Autodesk Inventor part; units mm, degrees
ref_plane "YZ Plane" through (0, 0, 0) normal (1, 0, 0) x (0, 1, 0)
ref_plane "XZ Plane" through (0, 0, 0) normal (0, 1, 0) x (-1, 0, 0)
ref_plane "XY Plane" through (0, 0, 0) normal (0, 0, 1) x (1, 0, 0)
sketch "Base" plane through (0, 0, 0) normal (0, 0, 1) x (1, 0, 0)
  circle A0 centre (0, 0) radius 19.125 construction
  arc A1 (28.5, 24.5) -> (24.5, 28.5) centre (24.5, 24.5) ccw
  line L0 (24.5, 28.5) -> (-24.5, 28.5)
  arc A2 (-24.5, 28.5) -> (-28.5, 24.5) centre (-24.5, 24.5) ccw
  line L1 (-28.5, 24.5) -> (-28.5, -24.5)
  arc A3 (-28.5, -24.5) -> (-24.5, -28.5) centre (-24.5, -24.5) ccw
  line L2 (-24.5, -28.5) -> (24.5, -28.5)
  arc A4 (24.5, -28.5) -> (28.5, -24.5) centre (24.5, -24.5) ccw
  line L3 (28.5, -24.5) -> (28.5, 24.5)
  circle A5 centre (-23.57, 23.57) radius 2
  circle A6 centre (23.57, 23.57) radius 2
  circle A7 centre (-23.57, -23.57) radius 2
  circle A8 centre (23.57, -23.57) radius 2
  circle A9 centre (0, 0) radius 20.125
  circle A10 centre (-17.9605, 17.9605) radius 2.489
  circle A11 centre (17.9605, -17.9605) radius 2.489
  point P0 (0, 0)
  dimension "d0" = 1
extrude "Plate1" add sketch "Base" along normal blind 2.54
sketch "Sketch2" plane through (0, 0, 2.54) normal (0, 0, 1) x (1, 0, 0)
  line L0 (28.5, -24.5) -> (28.5, 24.5)
  line L1 (28.5, -24.5) -> (28.5, -84.5)
  line L2 (-28.5, 24.5) -> (-28.5, -24.5)
  line L3 (-28.5, -24.5) -> (-28.5, -84.5)
  line L4 (28.5, -84.5) -> (-28.5, -84.5)
  arc A0 (24.5, -28.5) -> (28.5, -24.5) centre (24.5, -24.5) ccw
  line L5 (24.5, -28.5) -> (-24.5, -28.5)
  arc A1 (-28.5, -24.5) -> (-24.5, -28.5) centre (-24.5, -24.5) ccw
  point P0 (0, 0)
  dimension "d2" = 60
sheet face with bend "Face2" sketch "Sketch2" thickness 2.54 toward (0, 0, -1) bend radius 2.54
bend "Bend1"
sketch "Sketch3" plane through (28.5, -81.96, 0) normal (0, -1, 0) x (1, 0, 0)
  line L0 (-57, 0) -> (0, 0)
  line L1 (0, 0) -> (0, 25)
  line L2 (0, 25) -> (-57, 25)
  line L3 (-57, 25) -> (-57, 0)
edge flange "Flange1" height 25 angle 90 thickness 2.54 bend radius 2.54 thickness toward (0, -1, 0) relief tear relief width 2.54 relief depth 1.27 edges at (0, -84.5, 2.54) wall of the first edge with corners at (-28.5, -81.96, 0) (28.5, -81.96, 0) (28.5, -81.96, 25) (-28.5, -81.96, 25)
bend "Bend2"
corner "Corner1"
sketch "Sketch4" plane through (-28.5, -84.5, 25) normal (0, -1, 0) x (1, 0, 0)
  line L0 (0, 0) -> (57, 0) construction
  line L1 (28.5, 0) -> (28.5, -19.92) construction
  line L2 (57, -19.92) -> (0, -19.92) construction
  circle A0 centre (8, -8) radius 3
  circle A1 centre (49, -8) radius 3
  line L3 (0, -19.92) -> (0, 0)
  circle A2 centre (20.5, -8) radius 3
  circle A3 centre (36.5, -8) radius 3
  point P0 (28.5, -25)
  dimension "d18" = 6
  dimension "d19" = 8
  dimension "d20" = 8
  dimension "d21" = 8
  dimension "d22" = 8
  dimension "d25" = 12.5
extrude "Cut1" cut sketch "Sketch4" against normal blind 2.54
equation "\"d22\" = d19"
equation "\"d23\" = Thickness"
equation "\"d1\" = Thickness"
equation "\"d3\" = BendRadius"
equation "\"d4\" = BendReliefWidth"
equation "\"d6\" = MinimumRemnant"
equation "\"d5\" = BendReliefDepth"
equation "\"d7\" = TransitionRadius"
equation "\"d8\" = BendReliefWidth"
equation "\"d9\" = BendReliefDepth"
equation "\"d10\" = MinimumRemnant"
equation "\"d11\" = TransitionRadius"
equation "\"d14\" = BendRadius"
equation "\"d15\" = CornerReliefSize"
equation "\"d16\" = GapSize"
equation "\"d17\" = JacobiRadiusSize"
equation "\"BendRadius\" = Thickness"
equation "\"BendReliefWidth\" = Thickness"
equation "\"BendReliefDepth\" = 0.5 * Thickness"
equation "\"CornerReliefSize\" = 4 * Thickness"
equation "\"MinimumRemnant\" = 2 * Thickness"
equation "\"TransitionRadius\" = BendRadius"
equation "\"JacobiRadiusSize\" = BendRadius"
equation "\"GapSize\" = Thickness"
properties part number "NeckStepperCover"
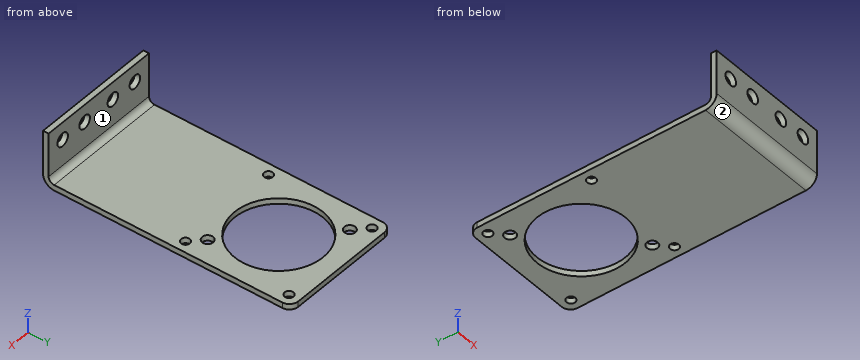
Read the model definition and answer for the solid it produces. Units are mm, in the model's axes. Face numbers are marked on the shaded views. A direction names the side the tool comes from. Give positions to 0.01 mm unless a question says otherwise; leave off trailing zeros. Order: outer loops, then holes, each group sorted by start corner. A loop starts at its lowest first (then second) coordinate and runs counter-clockwise, first axis right, second up.
(1) Find section D-D (x = -9.5). Give the vertices of the cut face in (y, z).
(2) Given pin 1 (1.5 mm diameter, centred on x = 20.5, y = -57, fed in from +Z); pin 2 (8 mm diameter, centred on x = 8, z = 17, fed in from +Y), each flat-ended and moving along its own axis, determine where each tip first touches the part or whether it passes through.
(3) Find section C-C (y = -23.57). Give the vertices of the cut face in (x, z), plus the area to 3 significant figures.
(4) Straight lines are drawn through the part: L1, parallel to Y at x = -2.5, z = 14.5; L2, parallel to Y at x = 23.57, z = 1.45; L3, parallel to Z at x = -18.5, y = -47.5. For each, find the intervals that lie inside material, in ascending order.
(5) For the marked faces 1 and 2, determine the directions among +Z, -Z, +X, -X, +Y, -Y from which every point of the face is accessible in a straight line to the end or side of a thin tool.
(6) Find section A-A (z = 17). Give the vertices of the cut face in (x, y).
(7) Find section B-B (x = 0). Give the vertices of the cut face in (y, z) (3 decimals).
Result sheet:
1. outline: (-84.5, 5.08) arc R5.08 ccw to (-79.42, 0) - (-17.74, 0) - (-17.74, 2.54) - (-79.42, 2.54) arc R2.54 cw to (-81.96, 5.08) - (-81.96, 14.4) - (-84.5, 14.4) - close; (-84.5, 19.6) - (-81.96, 19.6) - (-81.96, 25) - (-84.5, 25) - close; (17.74, 0) - (28.5, 0) - (28.5, 2.54) - (17.74, 2.54) - close
2. pin 1: stops at z = 2.54
2. pin 2: stops at y = -81.96
3. outline: (-28.5, 0) - (-25.57, 0) - (-25.57, 2.54) - (-28.5, 2.54) - close; (-21.57, 0) - (21.57, 0) - (21.57, 2.54) - (-21.57, 2.54) - close; (25.57, 0) - (28.5, 0) - (28.5, 2.54) - (25.57, 2.54) - close
3. area: 124 mm2
4. L1: y = -84.5 to -81.96
4. L2: y = -82.97 to -25.57, -21.57 to 21.57, 25.57 to 28.5
4. L3: z = 0 to 2.54
5. face 1: +Z, +X, -X, +Y
5. face 2: -Z, +X, -X, -Y
6. outline: (-28.5, -84.5) - (-23.5, -84.5) - (-23.5, -81.96) - (-28.5, -81.96) - close; (-17.5, -84.5) - (-11, -84.5) - (-11, -81.96) - (-17.5, -81.96) - close; (-5, -84.5) - (5, -84.5) - (5, -81.96) - (-5, -81.96) - close; (11, -84.5) - (17.5, -84.5) - (17.5, -81.96) - (11, -81.96) - close; (23.5, -84.5) - (28.5, -84.5) - (28.5, -81.96) - (23.5, -81.96) - close
7. outline: (-84.5, 5.08) arc R5.08 ccw to (-79.42, 0) - (-20.125, 0) - (-20.125, 2.54) - (-79.42, 2.54) arc R2.54 cw to (-81.96, 5.08) - (-81.96, 25) - (-84.5, 25) - close; (20.125, 0) - (28.5, 0) - (28.5, 2.54) - (20.125, 2.54) - close
